Work out the finished part from the listing and answer in its coordinate system (mm). A direction names the side the tool comes from. Round coordinates to 2 decimals unless told otherwise and drop trailing zeros. Loops run counter-clockwise (first coordinate to the right, second up) from the corner with the lowest first, then second, coordinate; pieces in that order, holes last. Notation, with made-up numbers: M 44,-39 L 69,-39 A21 ccw 69,-34 Z; hole C 69,9.5 d8. An arc over 180 degrees is marked long. One line per item, written item: value.
```python
from build123d import *

# Parameters (mm, degrees)
SKETCH_1_W      = 50
SKETCH_1_H      = 50
EXTRUDE_1_DEPTH = 30
FILLET_1_R      = 5
SKETCH_2_R      = 4
EXTRUDE_2_DEPTH = 100


with BuildPart() as part:
    # 草图1 → 凸台-拉伸1 (new body)
    with BuildSketch(Plane(origin=(0, 0, 0), x_dir=(1, 0, 0), z_dir=(0, 1, 0))):
        Rectangle(SKETCH_1_W, SKETCH_1_H)
    extrude(amount=EXTRUDE_1_DEPTH)

    # 圆角1
    fillet_1_edges = [part.edges().sort_by_distance(p)[0] for p in [
        (25, 30, 0),
        (0, 30, -25),
        (-25, 30, 0),
        (-25, 15, -25),
        (25, 15, -25),
        (25, 15, 25),
        (-25, 15, 25),
        (0, 30, 25),
    ]]
    fillet(fillet_1_edges, radius=FILLET_1_R)

    # 草图2 → 凸台-拉伸2 (add)
    with BuildSketch(Plane(origin=(0, 30, 0), x_dir=(1, 0, 0), z_dir=(0, 1, 0))):
        with Locations(Location((0, 0, 0), (0, 0, 270))):
            Circle(SKETCH_2_R)
    extrude(amount=EXTRUDE_2_DEPTH)

    # 草图3 → 旋转1 (revolve)
    with BuildSketch(Plane.XY):
        with BuildLine():
            Line((0, 130), (0, 128))
            ThreePointArc((0, 128), (12.5, 140.5), (0, 153))
            Line((0, 153), (0, 130))
        make_face()
    revolve(axis=Axis((0, 130, 0), (0, 1, 0)))


solid = part.part
```
1) Find the intervals of material crossed by probe 1 along X at (y, z) = (71, -0.5); probe 2 along Y at (x, z) = (-15.5, -4); probe 3 along Z at (x, y) = (-1, 100), in increasing order. Write a range as from..to.
Check values:
probe 1: -3.97..3.97
probe 2: 0..30
probe 3: -3.87..3.87
2) The mould has two halves that part along Y. Classify faces 1 (the face through (-24, 28, 0)), 2 (the face through (0, 12, 25)), 3 (the face through (4.2, 30, -0.3)): +Y half, -Y half, draft (parallel to the pull), parting line (faces both ways), or undercut.
Check values:
face 1: +Y half
face 2: draft
face 3: undercut
3) This flat-tipped pin is pushed along its axis until it touches: pin 1 (8 mm diameter, centred on y = 103.5, z = -1.5, fed in from -X). Where does it stop, or does it pass through?
Check values:
pin 1: x = -4
4) Find section A-A (x = 0). Give the vertices of the cut face in (y, z).
Check values:
outline: M 0,-25 L 25,-25 A5 ccw 30,-20 L 30,-4 L 128.66,-4 A12.5 ccw long 128.66,4 L 30,4 L 30,20 A5 ccw 25,25 L 0,25 Z
5) Find section B-B (z = 0). Give the vertices of the cut face in (x, y).
Check values:
outline: M -25,0 L 25,0 L 25,25 A5 ccw 20,30 L 4,30 L 4,128.66 A12.5 ccw long -4,128.66 L -4,30 L -20,30 A5 ccw -25,25 Z
6) Find section C-C (x = -9). Give the vertices of the cut face in (y, z).
Check values:
outline: M 0,-25 L 25,-25 A5 ccw 30,-20 L 30,20 A5 ccw 25,25 L 0,25 Z; C 140.5,0 d17.35
7) For faces 4 (the face through (0, 28, 24)), 5 (the face through (-3.905, 78.638, -0.867)), determine the directions among +Z, -Z, +X, -X, +Y, -Y from which every point of the face is accessible in a straight line to the end or side of a thin tool.
Check values:
face 4: +Z, +X, -X, +Y
face 5: none
8) Find section D-D (y = 77). Give the vertices of the cut face in (x, z).
Check values:
outline: C 0,0 d8
